Part print with two shaded views. Sizes in mm from the minimum x, y, z corner. Round coordinates to 2 decimals unless told otherwise and drop trailing zeros. Loops run counter-clockwise (first coordinate to the right, second up) from the corner with the lowest first, then second, coordinate; pieces in that order, holes last.
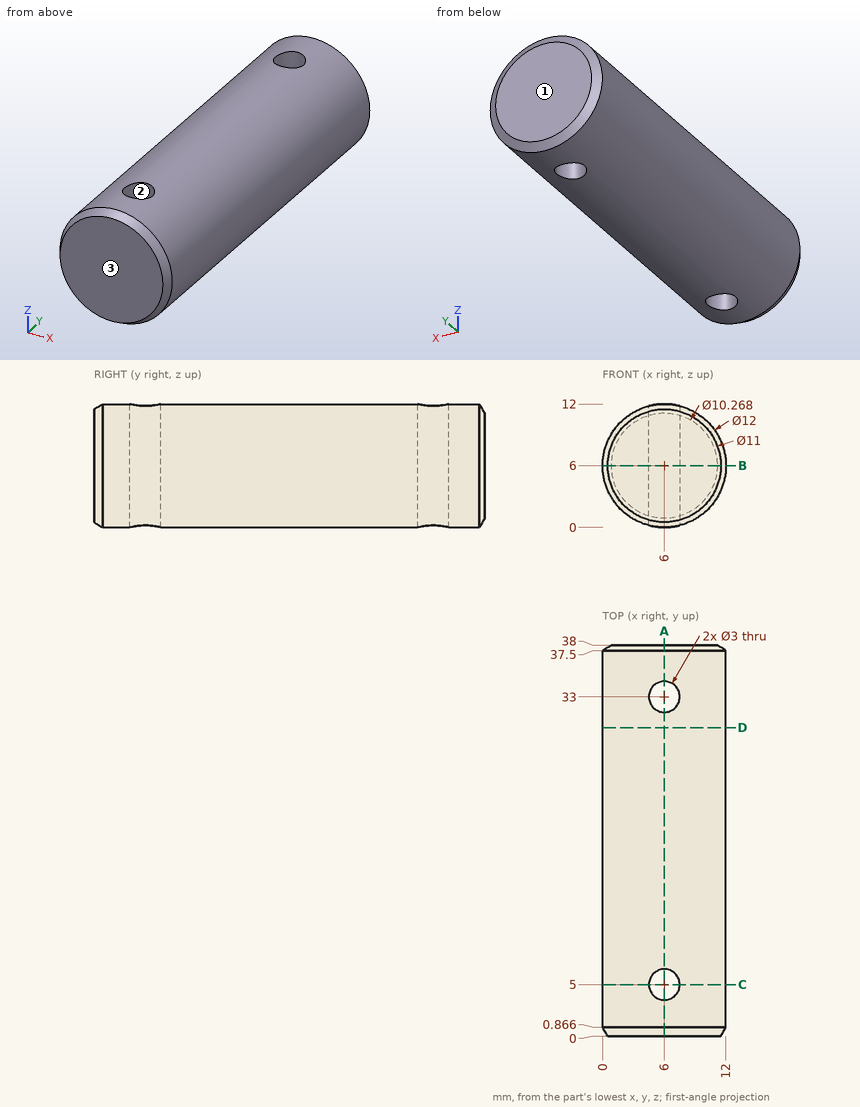
Item 1: Mould opens along Y. For the marked faces 1, 2 and 3 say: released by +Y, released by -Y, zero draft, split by the parting line, or undercut.
Verdict:
face 1: released by +Y
face 2: undercut
face 3: released by -Y
Item 2: Flat gauge pins, fed straight in: P1, Ø1.8, axis at x = 6, y = 5, coming from the -Z side; P2, Ø3, axis at x = 4, y = 19.5, coming from the -Z side; P3, Ø5, axis at x = 4, y = 24, coming from the +Z side; P4, Ø2, axis at y = 8.5, z = 7.5, coming from the -X side. Where does each tip first touch, or does it go through?
Verdict:
P1: passes through
P2: stops at z = 0.02
P3: stops at z = 12
P4: stops at x = 0.02
Item 3: Cut at C-C (y = 5). List the corners of the cut face in (x, z).
Verdict:
outline: (4.5, 0.19) - (4.5, 11.81) arc R6 ccw to start; (7.5, 0.19) arc R6 ccw to (7.5, 11.81) - close
Item 4: Cut at D-D (y = 30). List the corners of the cut face in (x, z), plus the area to 3 significant figures.
Verdict:
outline: circle Ø12 at (6, 6)
area: 113 mm2
Item 5: Cut at A-A (x = 6). List the corners of the cut face in (y, z).
Verdict:
outline: (0, 0.5) - (0.87, 0) - (3.5, 0) - (3.5, 12) - (0.87, 12) - (0, 11.5) - close; (6.5, 0) - (31.5, 0) - (31.5, 12) - (6.5, 12) - close; (34.5, 0) - (37.5, 0) - (38, 0.87) - (38, 11.13) - (37.5, 12) - (34.5, 12) - close
Item 6: Cut at B-B (z = 6). List the corners of the cut face in (x, y), plus the area to 3 significant figures.
Verdict:
outline: (0, 0.87) - (0.5, 0) - (11.5, 0) - (12, 0.87) - (12, 37.5) - (11.13, 38) - (0.87, 38) - (0, 37.5) - close; hole circle Ø3 at (6, 5); hole circle Ø3 at (6, 33)
area: 441 mm2
Item 7: Wall check: L1, parallel to X at y = 32, z = 9.5; L2, parallel to Y at x = 3.5, z = 10.5; L3, parallel to Y at x = 7.25, z = 10.25. Give the ranges that are in metal, low to high.
Verdict:
L1: x = 1.13 to 4.88, 7.12 to 10.87
L2: y = 0 to 37.99
L3: y = 0 to 4.17, 5.83 to 32.17, 33.83 to 38
